```python
from build123d import *

# Parameters (mm, degrees)
ESQUISSE1_R          = 5
BOSS_EXTRU_1_DEPTH   = 4
D_GAGEMENT_M82_D     = 10
D_GAGEMENT_M82_DEPTH = 222.5
D_GAGEMENT_M82_TIP   = 3.004303095


with BuildPart() as part:
    # Esquisse1 → Boss.-Extru.1 (new body)
    with BuildSketch(Plane.XY):
        with BuildLine():
            Line((-9.5, -12.5), (9.5, -12.5))
            ThreePointArc((9.5, -12.5), (11.621320344, -11.621320344), (12.5, -9.5))
            Line((12.5, -9.5), (12.5, 9.5))
            ThreePointArc((12.5, 9.5), (11.621320344, 11.621320344), (9.5, 12.5))
            Line((9.5, 12.5), (-9.5, 12.5))
            ThreePointArc((-9.5, 12.5), (-11.621320344, 11.621320344), (-12.5, 9.5))
            Line((-12.5, 9.5), (-12.5, -9.5))
            ThreePointArc((-12.5, -9.5), (-11.621320344, -11.621320344), (-9.5, -12.5))
        make_face()
        Circle(ESQUISSE1_R, mode=Mode.SUBTRACT)
    extrude(amount=BOSS_EXTRU_1_DEPTH)

    # Dégagement M82
    with Locations(Plane(origin=(0, -679.483503367, 39), x_dir=(1, 0, 0), z_dir=(0, 0, 1))):
        with Locations((0, 680), (0, 580), (0, 480)):
            Hole(D_GAGEMENT_M82_D / 2, depth=D_GAGEMENT_M82_DEPTH)
            with Locations((0, 0, -(D_GAGEMENT_M82_DEPTH + D_GAGEMENT_M82_TIP / 2))):  # 118° drill point
                Cone(0, D_GAGEMENT_M82_D / 2, D_GAGEMENT_M82_TIP, mode=Mode.SUBTRACT)


solid = part.part
```
Model file for the job. Use its own axes, mm. A direction names the side the tool comes from. Give positions to 0.01 mm unless a question says otherwise; leave off trailing zeros. Loops run counter-clockwise (first coordinate to the right, second up) from the corner with the lowest first, then second, coordinate; pieces in that order, holes last. Notation, with made-up numbers: (37.5, 6) -> (71.5, 6) arc R8 ccw to (71.5, 11) -> close; hole circle Ø10 at (44, -17.5). An arc over 180 degrees is marked (long way). Use CSV: the item, a comma, the result in double quotes. Start each with the question number.
1) Mould opens along Y. For faces 3 (the cylindrical face through (11.64, 11.6, 1.97)), 4 (the cylindrical face through (11.6, -11.64, 1.97)), 5 (the cylindrical face through (-0.114, 5.515, 1.972)) say: released by +Y, released by -Y, zero draft, split by the parting line, or undercut.
2) Slice it at B-B on y = 1.75. Give the cut face in (x, z).
3) Tool access for faces 1 (the cylindrical face through (0, -5, 2)), 2 (the flat face through (0, 12.5, 2)): list every direction of +Z, -Z, +X, -X, +Y, -Y with a clear straight run to the whole face (end or side of a thin tool).
4) Slice it at C-C on z = 0.6. Give the cut face in (x, y), plus the area to 3 significant figures.
5) Wall check: line 1 (X direction, y = 0, z = 0.5); line 2 (X direction, y = 4.25, z = 0.7); line 3 (X direction, y = 11.5, z = 2.2). Give the ranges that are in metal, low to high.
6) Slice it at A-A on x = 0. Give the cut face in (y, z).
Computed values:
1,face 3,"released by +Y"
1,face 4,"released by -Y"
1,face 5,"undercut"
2,outline,"(-12.5, 0) -> (-4.85, 0) -> (-4.85, 4) -> (-12.5, 4) -> close; (4.85, 0) -> (12.5, 0) -> (12.5, 4) -> (4.85, 4) -> close"
3,face 1,"+Z, -Z"
3,face 2,"+Z, -Z, +X, -X, +Y"
4,outline,"(-12.5, -9.5) arc R3 ccw to (-9.5, -12.5) -> (9.5, -12.5) arc R3 ccw to (12.5, -9.5) -> (12.5, 9.5) arc R3 ccw to (9.5, 12.5) -> (-9.5, 12.5) arc R3 ccw to (-12.5, 9.5) -> close; hole (-4.99, 0.26) arc R5 ccw (long way) to (4.99, 0.26) arc R5 ccw (long way) to start"
4,area,"534 mm^2"
5,line 1,"x = -12.5 to -5, 5 to 12.5"
5,line 2,"x = -12.5 to -3.33, 3.33 to 12.5"
5,line 3,"x = -11.74 to 11.74"
6,outline,"(-12.5, 0) -> (-5, 0) -> (-5, 4) -> (-12.5, 4) -> close; (5.52, 0) -> (12.5, 0) -> (12.5, 4) -> (5.52, 4) -> close"
